```python
from build123d import *

# Parameters (mm, degrees)
BOSS_EXTRUDE1_DEPTH         = 15.875
CUT_EXTRUDE1_DEPTH          = 152.4
F_1_4_0_25_DIAMETER_HOLE1_D = 3.96875
CUT_EXTRUDE2_DEPTH          = 11.43
SKETCH8_R                   = 4.1275
CUT_EXTRUDE3_DEPTH          = 5.08
FILLET1_R                   = 6.35


with BuildPart() as part:
    # Sketch1 → Boss-Extrude1 (new, symmetric)
    with BuildSketch(Plane.XY):
        Polygon((0, 0), (12.7, 0), (12.7, 25.4), (-12.7, 25.4), (-12.7, 0), align=None)
    extrude(amount=BOSS_EXTRUDE1_DEPTH, both=True)

    # Sketch2 → Cut-Extrude1 (cut)
    with BuildSketch(Plane.ZY.offset(12.7)):
        Polygon((0, 8.59506403), (-8.980256121, 17.575320151), (-10.102788136, 16.452788136), (0, 6.35), (10.102788136, 16.452788136), (8.980256121, 17.575320151), align=None)
    extrude(amount=-CUT_EXTRUDE1_DEPTH, mode=Mode.SUBTRACT)

    # 1/4 (0.25) Diameter Hole1 (through all)
    with Locations(Plane(origin=(0, 25.4, 0), x_dir=(1, 0, 0), z_dir=(0, 1, 0))):
        with Locations((0, 0), (76.2, 0)):
            Hole(F_1_4_0_25_DIAMETER_HOLE1_D / 2)

    # Sketch7 → Cut-Extrude2 (cut)
    with BuildSketch(Plane(origin=(0, 25.4, 0), x_dir=(1, 0, 0), z_dir=(0, 1, 0))):
        Polygon((5.132643893, 0), (2.566321947, 4.445), (-2.566321947, 4.445), (-5.132643893, 0), (-2.566321947, -4.445), (2.566321947, -4.445), align=None)
    extrude(amount=-CUT_EXTRUDE2_DEPTH, mode=Mode.SUBTRACT)

    # Sketch8 → Cut-Extrude3 (cut)
    with BuildSketch(Plane.XZ):
        with Locations(Location((0, 0, 0), (0, 0, 270))):
            Circle(SKETCH8_R)
    extrude(amount=-CUT_EXTRUDE3_DEPTH, mode=Mode.SUBTRACT)

    # Fillet1
    fillet1_edges = [part.edges().sort_by_distance(p)[0] for p in [
        (0, 25.4, 15.875),
        (0, 0, 15.875),
        (0, 25.4, -15.875),
        (0, 0, -15.875),
    ]]
    fillet(fillet1_edges, radius=FILLET1_R)


solid = part.part
```
Geometry: final body of the model. Coordinates: model frame, mm. A direction names the side the tool comes from. Round coordinates to 2 decimals unless told otherwise and drop trailing zeros. Write each loop counter-clockwise with the first axis right and the second up, starting at its lowest first coordinate (ties: lowest second). Pieces come first, ordered by that corner, then holes.
Item 1: Set-up query: faces 3 (the face through (0, 20, 4.445)), 4 (the face through (-0.178, 17.006, 9.549)), 5 (the face through (-0.178, 23.49, -14.064)), 6 (the face through (0.178, 1.811, 13.965)), 7 (the face through (-2, 5.08, 1)). Return all of +Z, -Z, +X, -X, +Y, -Y with unobstructed straight access to the full face (end or side cutting, diameter ignored); none if empty.
Item 2: Material intervals for L1, parallel to Z at x = 11.25, y = 9.25 (3 decimals); L2, parallel to Z at x = 0, y = 12.5 (3 decimals); L3, parallel to X at y = 2, z = 0, sorted ascending.
Item 3: Pin query (flat end, axial travel): P1, Ø1, axis at x = -7.5, z = 11, coming from the +Y side; P2, Ø2.5, axis at x = 1, y = 20.5, coming from the -Z side; P3, Ø2.5, axis at x = 0, z = 0, coming from the +Y side (3 decimals). Return the tip coordinate at first contact, or that it passes through.
Item 4: Section query B-B (z = -7.5). Return loops of the section in (x, y).
Item 5: Section query A-A (x = -7.5). Return loops of the section in (y, z) (3 decimals), plus the area to 3 significant figures.
Item 6: Mould query, pull axis X, two halves, no side actions, for faces 1 (the face through (-0.178, 13.148, 4.553)), 2 (the face through (2.2, 13.97, -0.1)). Classes: +X half, -X half, draft (parallel to the pull), parting line (faces both ways), or undercut.
Item 7: Section query C-C (y = 23.5). Return loops of the section in (x, z) (3 decimals), plus the area to 3 significant figures.
Completed:
1. face 3: +Y
1. face 4: +X, -X
1. face 5: -Z, +X, -X, +Y
1. face 6: +Z, +X, -X, -Y
1. face 7: -Y
2. L1: z = -15.875 to -2.9, -0.655 to 0.655, 2.9 to 15.875
2. L2: z = -15.875 to -6.15, -3.905 to -1.984, 1.984 to 3.905, 6.15 to 15.875
2. L3: x = -12.7 to -4.13, 4.13 to 12.7
3. P1: stops at y = 25.32
3. P2: stops at z = -15.87
3. P3: passes through
4. outline: (-12.7, 0) - (12.7, 0) - (12.7, 13.85) - (-12.7, 13.85) - close; (-12.7, 16.1) - (12.7, 16.1) - (12.7, 25.4) - (-12.7, 25.4) - close
5. outline: (0, -9.525) arc R6.35 ccw to (6.35, -15.875) - (19.05, -15.875) arc R6.35 ccw to (25.4, -9.525) - (25.4, 9.525) arc R6.35 ccw to (19.05, 15.875) - (6.35, 15.875) arc R6.35 ccw to (0, 9.525) - close; hole (6.35, 0) - (16.453, -10.103) - (17.575, -8.98) - (8.595, 0) - (17.575, 8.98) - (16.453, 10.103) - close
5. area: 729 mm2
6. face 1: draft
6. face 2: undercut
7. outline: (-12.7, -14.055) - (12.7, -14.055) - (12.7, 14.055) - (-12.7, 14.055) - close; hole (-5.133, 0) - (-2.566, -4.445) - (2.566, -4.445) - (5.133, 0) - (2.566, 4.445) - (-2.566, 4.445) - close
7. area: 646 mm2
